Autodesk Inventor part; units mm, degrees
ref_plane "YZ Plane" through (0, 0, 0) normal (1, 0, 0) x (0, 1, 0)
ref_plane "XZ Plane" through (0, 0, 0) normal (0, 1, 0) x (-1, 0, 0)
ref_plane "XY Plane" through (0, 0, 0) normal (0, 0, 1) x (1, 0, 0)
sketch "Sketch1" plane through (0, 0, 0) normal (1, 0, 0) x (0, 1, 0)
  line L0 (0, 0) -> (2.5, 0)
  line L1 (0, 0) -> (4, 0)
  line L2 (2.5, 0) -> (2.5, -7)
  line L3 (2.5, -7) -> (0, -7)
  line L4 (0, -7) -> (20, -7)
  line L5 (4, 0) -> (4, -7)
  line L6 (2.5, -7) -> (2.5, -41)
  line L7 (20, -7) -> (20, -11)
  line L8 (20, -11) -> (2.5, -11)
  line L9 (20, -7) -> (22.5, -7)
  line L10 (22.5, -7) -> (22.5, -11)
  line L11 (22.5, -11) -> (20, -11)
  line L12 (20, -11) -> (20, -7)
  line L13 (20, -7) -> (20, -11)
  line L14 (4, 0) -> (2.5, 0)
  line L15 (2.5, 0) -> (2.5, -11)
  line L16 (2.5, -11) -> (4, -11)
  line L17 (4, -11) -> (4, 0)
  line L18 (2.5, -11) -> (22.5, -11)
  line L19 (22.5, -11) -> (22.5, -7)
  line L20 (22.5, -7) -> (2.5, -7)
  line L21 (2.5, -7) -> (2.5, -11)
  line L22 (2.5, -11) -> (6.5, -11)
  line L23 (0, -7) -> (0, -105.9451)
  line L24 (2.5, -41) -> (25, -41)
  line L25 (0, -82) -> (2.5, -82)
  line L26 (0, -82) -> (4, -82)
  line L27 (2.5, -82) -> (2.5, -75)
  line L28 (2.5, -75) -> (0, -75)
  line L29 (0, -75) -> (20, -75)
  line L30 (4, -82) -> (4, -75)
  line L31 (20, -75) -> (20, -71)
  line L32 (20, -71) -> (2.5, -71)
  line L33 (20, -75) -> (22.5, -75)
  line L34 (22.5, -75) -> (22.5, -71)
  line L35 (22.5, -71) -> (20, -71)
  line L36 (20, -71) -> (20, -75)
  line L37 (20, -75) -> (20, -71)
  line L38 (4, -82) -> (2.5, -82)
  line L39 (2.5, -82) -> (2.5, -71)
  line L40 (2.5, -71) -> (4, -71)
  line L41 (4, -71) -> (4, -82)
  line L42 (2.5, -71) -> (22.5, -71)
  line L43 (22.5, -71) -> (22.5, -75)
  line L44 (22.5, -75) -> (2.5, -75)
  line L45 (2.5, -75) -> (2.5, -71)
  line L46 (2.5, -71) -> (6.5, -71)
  line L47 (2.5, -11) -> (6.5, -11)
  line L48 (6.5, -11) -> (6.5, -71)
  line L49 (6.5, -71) -> (2.5, -71)
  line L50 (2.5, -71) -> (2.5, -11)
  line L51 (6.5, -11) -> (9.5, -11)
  line L52 (9.5, -11) -> (9.5, -14)
  line L53 (9.5, -14) -> (6.5, -14)
  line L54 (6.5, -14) -> (6.5, -11)
  line L55 (6.5, -71) -> (9.5, -71)
  line L56 (9.5, -71) -> (9.5, -68)
  line L57 (9.5, -68) -> (6.5, -68)
  line L58 (6.5, -68) -> (6.5, -71)
  dimension "d1" = 2.5
  dimension "d2" = 4
  dimension "d3" = 7
  dimension "d4" = 20
  dimension "d5" = 34
  dimension "d9" = 4
  dimension "d12" = 2.5
  dimension "d13" = 4
  dimension "d55" = 22.5
  dimension "d56" = 4
  dimension "d80" = 3
  dimension "d81" = 3
  dimension "d82" = 3
  dimension "d83" = 3
revolve "Revolution2" add sketch "Sketch1" angle 360 about axis through (0, 0, -7) along (0, 0, -1) contours L1 L5 L4 L2 | L4 L17 L8 L6 | L4 L7 L8 L17 | L8 L48 L24 L6 | L9 L10 L11 L7 | L24 L48 L32 L50 | L8 L52 L53 L48 | L29 L30 L26 L27 | L39 L32 L41 L29 | L41 L32 L31 L29 | L57 L56 L32 L48 | L31 L35 L34 L33
sketch "Sketch6" plane through (0, 0, 0) normal (0, 1, 0) x (-1, 0, 0)
  line L0 (-2.5, -82) -> (2.5, -82)
  line L1 (0, -82) -> (0, -62)
  line L2 (0, -82) -> (20, -82) construction
  line L3 (0, -65) -> (15, -65) construction
  line L4 (0, -59) -> (15, -59) construction
  line L5 (10.6066, -48.3934) -> (10.6066, -54.3934)
  line L6 (0, -65) -> (0, -59)
  line L7 (0, -62) -> (0, -59.5)
  line L8 (0, -59.5) -> (10.6066, -48.8934)
  line L9 (10.6066, -48.8934) -> (10.6066, -53.8934)
  line L10 (10.6066, -53.8934) -> (0, -64.5)
  line L11 (0, -59.5) -> (0, -64.5)
  point P0 (0, 0)
  dimension "d64" = 20
  dimension "d65" = 90
  dimension "d69" = 15
  dimension "d71" = 15
  dimension "d75" = 2.5
  dimension "d76" = 5
extrude "Extrusion6" cut sketch "Sketch6" along normal mid plane 5
sketch "Sketch7" plane through (0, 0, 0) normal (0, 0, 1) x (1, 0, 0)
  arc A0 (-1.9966, -1.5104) -> (-1.9966, 1.4896) centre (0.0034, -0.0104) ccw
  line L0 (-1.9966, -0.0104) -> (-1.9966, 1.4896)
  line L1 (-1.9966, -0.0104) -> (-1.9966, -1.5104)
  line L2 (-1.9966, 1.4896) -> (-1.9966, -2.007)
  line L3 (-1.9966, -2.007) -> (-3.9862, -2.007)
  line L4 (-3.9862, -2.007) -> (-3.9862, 1.4896)
  line L5 (-3.9862, 1.4896) -> (-1.9966, 1.4896)
  line L6 (-1.9966, -1.5104) -> (-3.2272, -1.5104)
  line L7 (-3.2272, -1.5104) -> (-3.2272, 1.4896)
  line L8 (-3.2272, 1.4896) -> (-1.9966, 1.4896)
  line L9 (-1.9966, 1.4896) -> (-1.9966, -1.5104)
  point P0 (0, 0)
  point P1 (0, 0)
  dimension "d77" = 5
extrude "Extrusion7" add sketch "Sketch7" against normal blind 26 contours L6 L7 L5 L0 L1
sketch "Sketch8" plane through (0, 0, -14) normal (0, 0, -1) x (-1, 0, 0)
  circle A0 centre (0, 0) radius 6.5
  dimension "d84" = 13
extrude "Extrusion8" cut sketch "Sketch8" against normal blind 4
sketch "Sketch9" plane through (0, 0, -14) normal (0, 0, -1) x (-1, 0, 0)
  circle A0 centre (0, 0) radius 22.5
extrude "Extrusion9" cut sketch "Sketch9" along normal blind 400
sketch "Sketch10" plane through (0, 0, -14) normal (0, 0, -1) x (-1, 0, 0)
  circle A0 centre (0, 0) radius 9.5
  circle A1 centre (0, 0) radius 6.5
extrude "Extrusion10" cut sketch "Sketch10" against normal blind 5
sketch "Sketch11" plane through (0, 0, -10) normal (0, 0, -1) x (-1, 0, 0)
  circle A0 centre (0, 0) radius 5
  circle A1 centre (0, 0) radius 4
  circle A2 centre (0, 0) radius 2.5
  arc A3 (2.0077, 1.4896) -> (1.9966, -1.5045) centre (0, 0) ccw
  line L0 (1.9966, -1.5045) -> (3.0554, -1.5045)
  line L1 (3.0554, -1.5045) -> (3.0554, 1.7409)
  line L2 (3.0554, 1.7409) -> (1.9966, 1.7409)
  line L3 (1.9966, 1.7409) -> (1.9966, -1.5045)
  dimension "d91" = 10
  dimension "d92" = 5
extrude "Extrusion11" add sketch "Sketch11" along normal blind 10 contours A0 | A1 | A2 L3 | A2 L3 L2 L1 L0 picked at (2.0884, -0.3478)
sketch "Sketch12" plane through (0, 0, -9) normal (0, 0, -1) x (-1, 0, 0)
  circle A0 centre (0, 0) radius 5
  circle A1 centre (0, 0) radius 9.5
extrude "Extrusion12" add sketch "Sketch12" along normal blind 2
sketch "Sketch13" plane through (0, 0, -11) normal (0, 0, -1) x (-1, 0, 0)
  circle A0 centre (0, 0) radius 5
  circle A1 centre (0, 0) radius 6
  dimension "d97" = 12
extrude "Extrusion13" cut sketch "Sketch13" against normal blind 1
sketch "Sketch14" plane through (0, 0, -11) normal (0, 0, -1) x (-1, 0, 0)
  circle A0 centre (0, 0) radius 5
  circle A1 centre (0, 0) radius 6
  circle A2 centre (0, 0) radius 7.5
  dimension "d100" = 15
extrude "Extrusion14" add sketch "Sketch14" along normal blind 5 contours A2
sketch "Sketch15" plane through (-1.9966, -1.5045, 0) normal (1, 0, 0) x (0, 0, -1)
  line L0 (20, 0) -> (20, 3.009)
  line L1 (20, 1.5045) -> (0, 1.5045)
  line L2 (20, 1.5045) -> (17.5, 1.5045)
  line L3 (15.9505, 1.5045) -> (13.4505, 1.5045)
  circle A0 centre (13.4505, 1.5045) radius 1.5
  dimension "d103" = 2.5
  dimension "d104" = 2.5
  dimension "d105" = 3
extrude "Extrusion15" cut sketch "Sketch15" against normal blind 20
properties part number "Spool_revB2"
Can you work these out from the model? Positions are in its coordinate system, mm. A direction names the side the tool comes from. Round coordinates to 2 decimals unless told otherwise and drop trailing zeros. Write each loop counter-clockwise with the first axis right and the second up, starting at its lowest first coordinate (ties: lowest second). Pieces come first, ordered by that corner, then holes. Notation, with made-up numbers: (16.5, 66) - (25.5, 66) arc R23 ccw to (25.5, 103) - close; hole circle Ø2 at (-3.5, 76.25). An arc over 180 degrees is marked (long way). Write each question's results on one line, items separated by ' | '. Start each with the question number.
1) Suppose I cut it at B-B (y = 0). Give the number of separate pieces and of enclosed holes in the cut face, and give its area (3 significant figures).
2) Suppose I cut it at A-A (x = 0). List the corners of the cut face in (y, z) for me.
3) Suppose I cut it at D-D (y = 18). List the corners of the cut face in (x, z) for me.
4) We'd pull the mould along X, two halves only. Please class faces 6 (the flat face through (-1.997, 0, -10)), 7 (the cylindrical face through (-19.961, 10.382, -9.028)), 8 (the flat face through (-2, 6, -16)): released by +X, released by -X, zero draft, split by the parting line, or undercut.
5) Which directions (+Z, -Z, +X, -X, +Y, -Y) give clear straight access to the entire face, cutting with the end or side of a thin tool? Please do faces 1 (the cylindrical face through (1.08, 4.88, -14.93)), 2 (the cylindrical face through (-3.905, -0.867, -3.549)), 3 (the flat face through (2, 2, 0)), 4 (the cylindrical face through (-3.48, -0.57, -14.84)), 5 (the flat face through (-2.2, 0.1, -20)).
6) Please list where these lines run through material, in increasing order: line 1 (X direction, y = 0, z = -6.5); line 2 (Y direction, x = 0, z = -12.5); line 3 (Z direction, x = -7, y = 0).
7) For pin 1 Ø1.5 at (x, z) = (2.5, -15.5) entering from +Y; pin 2 Ø6 at (x, y) = (-11.5, -4) entering from -Z; pin 3 Ø3.5 at (y, z) = (0, -13.45) entering from -X, each with a flat end and sliding along its axis, tell me the tip position at first contact or that it passes through.
Here are the results:
1) separate pieces: 4 | enclosed holes: 0 | area: 236 mm2
2) outline: (-22.5, -11) - (-7.5, -11) - (-7.5, -16) - (-6, -16) - (-6, -10) - (-5, -10) - (-5, -20) - (-2.5, -20) - (-2.5, 0) - (-4, 0) - (-4, -7) - (-22.5, -7) - close; (2.5, -20) - (5, -20) - (5, -10) - (6, -10) - (6, -16) - (7.5, -16) - (7.5, -11) - (22.5, -11) - (22.5, -7) - (4, -7) - (4, 0) - (2.5, 0) - close
3) outline: (-13.5, -11) - (13.5, -11) - (13.5, -7) - (-13.5, -7) - close
4) face 6: undercut | face 7: split by the parting line | face 8: zero draft
5) face 1: -Z | face 2: +Z | face 3: +Z, +X, -X, +Y, -Y | face 4: -X | face 5: -Z, +X, -X, +Y, -Y
6) line 1: x = -4 to -2, 2.5 to 4 | line 2: y = -7.5 to -6, -5 to -2.5, 2.5 to 5, 6 to 7.5 | line 3: z = -16 to -14.95, -11.95 to -7
7) pin 1: stops at y = 7.29 | pin 2: stops at z = -11 | pin 3: stops at x = -7.5
